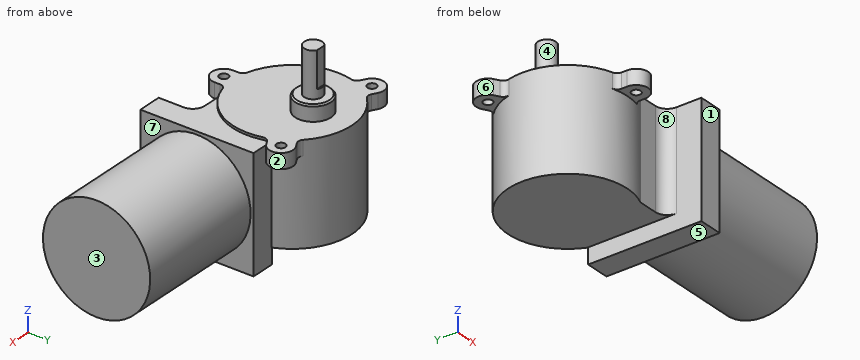
from build123d import *

# Parameters (mm, degrees)
SKETCH_1_R                       = 6
EXTRUDE_1_DEPTH                  = 5.2
CHAMFER_1_SIZE                   = 0.5
SKETCH_2_R                       = 3
EXTRUDE_2_DEPTH                  = 15
SKETCH_3_OUTSIDE_W               = 19.276
SKETCH_3_OUTSIDE_H               = 19.276
CUT_EXTRUDE_1_DEPTH              = 12
SKETCH_4_R                       = 20
EXTRUDE_3_DEPTH                  = 33.5
SKETCH_5_R                       = 1.5
EXTRUDE_4_DEPTH                  = 5
FILLET_2_R                       = 2
PATTERN_CIRCULAR_1_COUNT         = 3
FILLET_2_OF_PATTERN_CIRCULAR_1_R = 2
SKETCH_7_W                       = 38
SKETCH_7_H                       = 38
EXTRUDE_5_DEPTH                  = 8
EXTRUDE_6_REACH                  = 70.746
EXTRUDE_6_END_RADIUS             = 20
SKETCH_8_W                       = 32.7
SKETCH_8_H                       = 10.700657923
SKETCH_10_R                      = 18
EXTRUDE_7_DEPTH                  = 44
FILLET_1_R                       = 4


with BuildPart() as part:
    # ｽｹｯﾁ1 → ﾎﾞｽ - 押し出し1 (new body)
    with BuildSketch(Plane.XY):
        Circle(SKETCH_1_R)
    extrude(amount=EXTRUDE_1_DEPTH)

    # 面取り1
    chamfer_1_edges = [part.edges().sort_by_distance(p)[0] for p in [
        (-6, 0, 5.2),
    ]]
    chamfer(chamfer_1_edges, length=CHAMFER_1_SIZE)

    # ｽｹｯﾁ2 → ﾎﾞｽ - 押し出し2 (add)
    with BuildSketch(Plane.XY.offset(5.2)):
        Circle(SKETCH_2_R)
    extrude(amount=EXTRUDE_2_DEPTH)

    # ｽｹｯﾁ3 outside → ｶｯﾄ - 押し出し1 (cut)
    with BuildSketch(Plane.XY.offset(20.2)):
        Rectangle(SKETCH_3_OUTSIDE_W, SKETCH_3_OUTSIDE_H)
        with BuildLine():
            Line((-1.658312395, 2.5), (1.658312395, 2.5))
            ThreePointArc((1.658312395, 2.5), (0, -3), (-1.658312395, 2.5))
        make_face(mode=Mode.SUBTRACT)
    extrude(amount=-CUT_EXTRUDE_1_DEPTH, mode=Mode.SUBTRACT)

    # ｽｹｯﾁ4 → ﾎﾞｽ - 押し出し3 (add)
    with BuildSketch(Plane(origin=(0, 0, 0), x_dir=(-1, 0, 0), z_dir=(0, 0, -1))):
        with Locations((0, -7)):
            Circle(SKETCH_4_R)
    extrude(amount=EXTRUDE_3_DEPTH)

    # ｽｹｯﾁ5 → ﾎﾞｽ - 押し出し4 (add)
    with BuildSketch(Plane.XY):
        with BuildLine():
            Line((-4, -26.595917942), (-4, -30))
            ThreePointArc((-4, -30), (0, -34), (4, -30))
            Line((4, -30), (4, -26.595917942))
            Line((4, -26.595917942), (-4, -26.595917942))
        make_face()
        with Locations((0, -30)):
            Circle(SKETCH_5_R, mode=Mode.SUBTRACT)
    extrude_4 = extrude(amount=-EXTRUDE_4_DEPTH)

    # ﾌｨﾚｯﾄ2
    fillet_2_edges = [part.edges().sort_by_distance(p)[0] for p in [
        (-4, -26.595917942, -2.5),
        (4, -26.595917942, -2.5),
    ]]
    fillet(fillet_2_edges, radius=FILLET_2_R)

    # 円形ﾊﾟﾀｰﾝ1: ﾎﾞｽ - 押し出し4 ×3 about axis
    pattern_circular_1_axis = Axis((0, -7, 0), (0, 0, 1))
    for i in range(1, PATTERN_CIRCULAR_1_COUNT):
        add(extrude_4.rotate(pattern_circular_1_axis, i * 360 / PATTERN_CIRCULAR_1_COUNT))

    # ﾌｨﾚｯﾄ2 of 円形ﾊﾟﾀｰﾝ1
    fillet_2_of_pattern_circular_1_edges = [part.edges().sort_by_distance(p)[0] for p in [
        (18.970562748, -0.666142644, -2.5),
        (14.970562748, 6.262060586, -2.5),
        (-14.970562748, 6.262060586, -2.5),
        (-18.970562748, -0.666142644, -2.5),
    ]]
    fillet(fillet_2_of_pattern_circular_1_edges, radius=FILLET_2_OF_PATTERN_CIRCULAR_1_R)

    # ｽｹｯﾁ7 → ﾎﾞｽ - 押し出し5 (add)
    with BuildSketch(Plane(origin=(26.5, 0, 0), x_dir=(0, 0, -1), z_dir=(1, 0, 0))):
        with Locations((19.8, -18.7)):
            Rectangle(SKETCH_7_W, SKETCH_7_H)
    extrude(amount=-EXTRUDE_5_DEPTH)

    # ﾎﾞｽ - 押し出し6: up to this cylinder (the profile starts outside it)
    extrude_6_end = Plane(origin=(0, -7, -17.15), z_dir=(0, 0, 1)) * Cylinder(EXTRUDE_6_END_RADIUS, 182.492, mode=Mode.PRIVATE)
    # ｽｹｯﾁ8 → ﾎﾞｽ - 押し出し6 (add, up to the surface)
    with BuildSketch(Plane.ZY.offset(-18.5), mode=Mode.PRIVATE) as extrude_6_sk1:
        with Locations((-17.15, -19.949671039)):
            Rectangle(SKETCH_8_W, SKETCH_8_H)
    extrude_6_tool1 = extrude(extrude_6_sk1.sketch, amount=EXTRUDE_6_REACH, mode=Mode.PRIVATE) - extrude_6_end
    add(extrude_6_tool1.solids().sort_by_distance((18.5, -19.949671, -17.15))[0])

    # ｽｹｯﾁ10 → ﾎﾞｽ - 押し出し7 (add)
    with BuildSketch(Plane(origin=(26.5, 0, 0), x_dir=(0, 0, -1), z_dir=(1, 0, 0))):
        with Locations((19.8, -18.7)):
            Circle(SKETCH_10_R)
    extrude(amount=EXTRUDE_7_DEPTH)

    # ﾌｨﾚｯﾄ1
    fillet_1_edges = [part.edges().sort_by_distance(p)[0] for p in [
        (18.5, -25.3, -17.15),
    ]]
    fillet(fillet_1_edges, radius=FILLET_1_R)


solid = part.part
Source: CAD feature listing. Evaluate the final solid. Frame: model axes, mm. Face numbers are marked on the shaded views. A direction names the side the tool comes from. Coordinates: 2 decimals unless noted, no trailing zeros. Write each loop counter-clockwise with the first axis right and the second up, starting at its lowest first coordinate (ties: lowest second). Pieces come first, ordered by that corner, then holes. Notation, with made-up numbers: M 86.25,54.25 L 105.25,54.25 A18 cw 105.25,88.25 Z; hole C 19.25,18.25 d2. An arc over 180 degrees is marked long. Use a Markdown table: item, result.
1) Ray query, L1, parallel to Y at x = 0, z = -2.3; L2, parallel to Z at x = -4, y = -20; L3, parallel to Y at x = 14.5, z = -6. Return the intervals inside material, ascending.
Conclusion:
| item | result |
|---|---|
| L1 | y = -34 to -31.5, -28.5 to 13 |
| L2 | z = -33.5 to 0 |
| L3 | y = -25.3 to 6.77 |
2) Section B-B, the plane y = -18.7. Output: boundary loops of the cut face in (x, z).
Conclusion:
| item | result |
|---|---|
| outline | M -16.22,-33.5 L 18.5,-33.5 L 18.5,-38.8 L 26.5,-38.8 L 26.5,-37.8 L 70.5,-37.8 L 70.5,-1.8 L 26.5,-1.8 L 26.5,-0.8 L 16.22,-0.8 L 16.22,0 L -16.22,0 Z |
3) Section A-A, the plane x = 0. Output: boundary loops of the cut face in (y, z), then the cut area to 3 significant figures.
Conclusion:
| item | result |
|---|---|
| outline | M -34,-5 L -31.5,-5 L -31.5,0 L -34,0 Z; M -28.5,-5 L -27,-5 L -27,-33.5 L 13,-33.5 L 13,0 L 6,0 L 6,4.7 L 5.5,5.2 L 3,5.2 L 3,8.2 L 2.5,8.2 L 2.5,20.2 L -3,20.2 L -3,5.2 L -5.5,5.2 L -6,4.7 L -6,0 L -28.5,0 Z |
| area | 1,510 mm^2 |
4) Section D-D, the plane x = -15. Output: boundary loops of the cut face in (y, z).
Conclusion:
| item | result |
|---|---|
| outline | M -20.23,-33.5 L 6.23,-33.5 L 6.23,-5 L 6.81,-5 L 6.81,0 L -20.23,0 Z |
5) First-contact query: pin 1 Ø7 at (x, z) = (12.5, -17) entering from -Y; pin 2 Ø5.5 at (x, y) = (20.5, -15) entering from +Z; pin 3 Ø3.5 at (x, y) = (0, -30) entering from -Z. Flat tips, straight axial feed; report the tip coordinate or a pass-through.
Conclusion:
| item | result |
|---|---|
| pin 1 | stops at y = -25.59 |
| pin 2 | stops at z = 0 |
| pin 3 | stops at z = -5 |
6) Reachability of the marked faces 4, 5, 6, 7 and 8 from +Z, -Z, +X, -X, +Y, -Y: full face, straight path, thin tool, end or side. Return the list, or none.
Conclusion:
| item | result |
|---|---|
| face 4 | +Z |
| face 5 | -Z, +X, -X, +Y, -Y |
| face 6 | +Z, -Z |
| face 7 | +X |
| face 8 | +Z, -Z, -Y |
7) Section C-C, the plane z = -19.8. Output: boundary loops of the cut face in (x, y).
Conclusion:
| item | result |
|---|---|
| outline | M 8.07,-25.3 L 14.5,-25.3 A4 cw 18.5,-29.3 L 18.5,-37.7 L 26.5,-37.7 L 26.5,-36.7 L 70.5,-36.7 L 70.5,-0.7 L 26.5,-0.7 L 26.5,0.3 L 18.62,0.3 A20 ccw long Z |
8) Mould query, pull axis Y, two halves, no side actions, for the marked faces 1, 2 and 3. Classes: pulls with the +Y half, pulls with the -Y half, needs draft (parallel to the pull), parting line crosses it, or undercut.
Conclusion:
| item | result |
|---|---|
| face 1 | pulls with the -Y half |
| face 2 | undercut |
| face 3 | needs draft |
